```python
from build123d import *

# Parameters (mm, degrees)
EXTRUDE_1_DEPTH          = 3
EXTRUDE_2_DEPTH          = 287
SKETCH_4_W               = 21.736589458
SKETCH_4_H               = 200
CUT_EXTRUDE_1_DEPTH      = 43
SKETCH_5_W               = 23.415155123
SKETCH_5_H               = 200
CUT_EXTRUDE_2_DEPTH      = 43
CUT_EXTRUDE_6_DEPTH      = 100
CUT_EXTRUDE_6_DEPTH_BACK = 100
SKETCH_6_W               = 303.843563536
SKETCH_6_H               = 206
HOLE_WIZARD_1_AT_2_COUNT = 2
HOLE_WIZARD_1_AT_2_PITCH = 10
HOLE_WIZARD_1_AT_3_COUNT = 2
HOLE_WIZARD_1_AT_3_PITCH = 31.622776602
HOLE_WIZARD_1_AT_4_COUNT = 2
HOLE_WIZARD_1_AT_4_PITCH = 30
CUT_EXTRUDE_7_DEPTH      = 30


with BuildPart() as part:
    # 草图1 → 凸台-拉伸1 (new body)
    with BuildSketch(Plane.XY):
        Polygon((-143.75, 30), (-143.75, 70), (-105.75, 70), (-105.75, 65), (-100.25, 65), (-100.25, 70), (99.75, 70), (99.75, 65), (105.25, 65), (105.25, 70), (143.25, 70), (143.25, 30), (135.25, 30), (135.25, -30), (143.25, -30), (143.25, -70), (105.25, -70), (105.25, -65), (99.75, -65), (99.75, -70), (-100.25, -70), (-100.25, -65), (-105.75, -65), (-105.75, -70), (-143.75, -70), (-143.75, -30), (-135.75, -30), (-135.75, 30), align=None)
    extrude(amount=EXTRUDE_1_DEPTH)

    # 草图2 → 凸台-拉伸2 (add)
    with BuildSketch(Plane.ZY.offset(143.75)):
        with BuildLine():
            Line((0, 70), (0, 30))
            Line((0, 30), (-3, 33))
            Line((-3, 33), (-3, 70))
            ThreePointArc((-3, 70), (6.665476221, 93.334523779), (30, 103))
            Line((30, 103), (47, 103))
            Line((47, 103), (50, 100))
            Line((50, 100), (45, 90))
            Line((45, 90), (60, 90))
            Line((60, 90), (60, 87))
            Line((60, 87), (41, 87))
            Line((41, 87), (47, 100))
            Line((47, 100), (30, 100))
            ThreePointArc((30, 100), (8.786796564, 91.213203436), (0, 70))
        make_face()
        with BuildLine():
            Line((30, -100), (47, -100))
            Line((47, -100), (41, -87))
            Line((41, -87), (60, -87))
            Line((60, -87), (60, -90))
            Line((60, -90), (45, -90))
            Line((45, -90), (50, -100))
            Line((50, -100), (47, -103))
            Line((47, -103), (30, -103))
            ThreePointArc((30, -103), (6.665476221, -93.334523779), (-3, -70))
            Line((-3, -70), (-3, -33))
            Line((-3, -33), (0, -30))
            Line((0, -30), (0, -70))
            ThreePointArc((0, -70), (8.786796564, -91.213203436), (30, -100))
        make_face()
    extrude(amount=-EXTRUDE_2_DEPTH)

    # 草图4 → 切除-拉伸1 (cut)
    with BuildSketch(Plane.ZY.offset(143.75)):
        with Locations((49.368294729, 0)):
            Rectangle(SKETCH_4_W, SKETCH_4_H)
    extrude(amount=-CUT_EXTRUDE_1_DEPTH, mode=Mode.SUBTRACT)

    # 草图5 → 切除-拉伸2 (cut)
    with BuildSketch(Plane(origin=(143.25, 0, 0), x_dir=(0, 0, -1), z_dir=(1, 0, 0))):
        with Locations((-51.459603014, 0)):
            Rectangle(SKETCH_5_W, SKETCH_5_H)
    extrude(amount=-CUT_EXTRUDE_2_DEPTH, mode=Mode.SUBTRACT)

    # 草图6 → 切除-拉伸6 (cut, two sides: drawn at the far end of the back side and taken through both)
    with BuildSketch(Plane.XY.offset(-CUT_EXTRUDE_6_DEPTH_BACK)):
        with Locations((51.171781768, 0)):
            Rectangle(SKETCH_6_W, SKETCH_6_H)
    extrude(amount=CUT_EXTRUDE_6_DEPTH + CUT_EXTRUDE_6_DEPTH_BACK, mode=Mode.SUBTRACT)

    # 草图8 → 大小六角凹头盖螺钉柱孔1 (revolve, cut)
    with BuildSketch(Plane(origin=(-115.75, 15, 0), x_dir=(0, 1, 0), z_dir=(1, 0, 0))):
        Polygon((0, 0), (0, 50), (1.2, 50), (1.2, 2), (2.15, 2), (2.15, 0.024142219), (2.175, 0), align=None)
    hole_wizard_1 = revolve(axis=Axis((-115.75, 15, -6.35), (0, 0, 1)), mode=Mode.SUBTRACT)

    # 大小六角凹头盖螺钉柱孔1 at 2: 大小六角凹头盖螺钉柱孔1 ×2
    with Locations(*[(-i * HOLE_WIZARD_1_AT_2_PITCH, 0, 0) for i in range(1, HOLE_WIZARD_1_AT_2_COUNT)]):
        add(hole_wizard_1, mode=Mode.SUBTRACT)

    # 大小六角凹头盖螺钉柱孔1 at 3: 大小六角凹头盖螺钉柱孔1 ×2
    with Locations(*[Vector(-0.3162277660168408, -0.9486832980505129, 0) * (i * HOLE_WIZARD_1_AT_3_PITCH) for i in range(1, HOLE_WIZARD_1_AT_3_COUNT)]):
        add(hole_wizard_1, mode=Mode.SUBTRACT)

    # 大小六角凹头盖螺钉柱孔1 at 4: 大小六角凹头盖螺钉柱孔1 ×2
    with Locations(*[(0, -i * HOLE_WIZARD_1_AT_4_PITCH, 0) for i in range(1, HOLE_WIZARD_1_AT_4_COUNT)]):
        add(hole_wizard_1, mode=Mode.SUBTRACT)

    # 草图10 → 切除-拉伸7 (cut)
    with BuildSketch(Plane.ZY.offset(135.75)):
        with BuildLine():
            Line((30, 100), (47, 100))
            Line((47, 100), (45.5, 101.5))
            Line((45.5, 101.5), (30, 101.5))
            ThreePointArc((30, 101.5), (7.726136393, 92.273863607), (-1.5, 70))
            Line((-1.5, 70), (-1.5, 37.5))
            Line((-1.5, 37.5), (3, 33))
            Line((3, 33), (3, 70))
            Line((3, 70), (0, 70))
            ThreePointArc((0, 70), (8.786796564, 91.213203436), (30, 100))
        make_face()
        with BuildLine():
            Line((-1.5, -37.5), (-1.5, -70))
            ThreePointArc((-1.5, -70), (7.726136393, -92.273863607), (30, -101.5))
            Line((30, -101.5), (45.5, -101.5))
            Line((45.5, -101.5), (47, -100))
            Line((47, -100), (30, -100))
            ThreePointArc((30, -100), (8.786796564, -91.213203436), (0, -70))
            Line((0, -70), (3, -70))
            Line((3, -70), (3, -33))
            Line((3, -33), (-1.5, -37.5))
        make_face()
    extrude(amount=-CUT_EXTRUDE_7_DEPTH, mode=Mode.SUBTRACT)


solid = part.part
```
Geometry check sheet. Reference: the model listing, model coordinates, mm. A direction names the side the tool comes from. Round coordinates to 2 decimals unless told otherwise and drop trailing zeros. Write each loop counter-clockwise with the first axis right and the second up, starting at its lowest first coordinate (ties: lowest second). Pieces come first, ordered by that corner, then holes. Notation, with made-up numbers: (20, 81) -> (55, 81) arc R23 cw to (55, 119) -> close; hole circle Ø4 at (-1.75, 64). An arc over 180 degrees is marked (long way). Put each result on its own line as item: value.
1) Release check for a two-part mould opening along X. For faces 1 (the face through (-103, 68, 0)), 2 (the face through (-114, -15, 2)), 3 (the face through (-143.75, 69, 2)) record: pulls with the +X half, pulls with the -X half, needs draft (parallel to the pull), parting line crosses it, or undercut.
Recorded:
face 1: needs draft
face 2: undercut
face 3: pulls with the -X half
2) Thickness scan on probe 1 along X at (y, z) = (-15, 2.45); probe 2 along X at (y, z) = (15, 1.25); probe 3 along Y at (x, z) = (-120, 43.5). Record the ranges inside material, lowest first. Write a range as from..to.
Recorded:
probe 1: x = -135.75..-126.95, -124.55..-116.95, -114.55..-100.75
probe 2: x = -135.75..-127.9, -123.6..-117.9, -113.6..-100.75
probe 3: y = -103..-101.5, 101.5..103
3) Cross-section at B-B, the plane z = 35. Enter the section's corners in (x, y).
Recorded:
outline: (-143.75, -103) -> (-100.75, -103) -> (-100.75, -100) -> (-105.75, -100) -> (-105.75, -101.5) -> (-135.75, -101.5) -> (-135.75, -100) -> (-143.75, -100) -> close; (-143.75, 100) -> (-135.75, 100) -> (-135.75, 101.5) -> (-105.75, 101.5) -> (-105.75, 100) -> (-100.75, 100) -> (-100.75, 103) -> (-143.75, 103) -> close
4) Depth check by flat-ended pin: P1, Ø3.5, axis at x = -125.75, y = -15, coming from the +Z side; P2, Ø8, axis at x = -122.5, z = 23.5, coming from the -Y side; P3, Ø7, axis at x = -125.75, y = 15, coming from the -Z side; P4, Ø6, axis at y = -81.5, z = 7, coming from the -X side. Enter the tip coordinate at first touch or a pass-through.
Recorded:
P1: stops at z = 3
P2: stops at y = -102.91
P3: stops at z = 0
P4: passes through
5) Cross-section at A-A, the plane x = -139. Enter the section's corners in (y, z), plus the area to 3 significant figures.
Recorded:
outline: (-103, 30) arc R33 ccw to (-70, -3) -> (-33, -3) -> (-30, 0) -> (-30, 3) -> (-70, 3) -> (-70, 0) arc R30 cw to (-100, 30) -> (-100, 50) -> (-103, 47) -> close; (30, 0) -> (33, -3) -> (70, -3) arc R33 ccw to (103, 30) -> (103, 47) -> (100, 50) -> (100, 30) arc R30 cw to (70, 0) -> (70, 3) -> (30, 3) -> close
area: 879 mm2
6) Access from +Z, -Z, +X, -X, +Y, -Y to the whole of each face (thin tool, end or side, straight path). Record for faces 4 (the face through (-122.551, 93.077, 6.41)), 5 (the face through (-135.75, 67, 1)), 6 (the face through (-139.806, -90.979, 8.555)), 7 (the face through (-123.65, -15.47, 1)), 8 (the face through (-121, -54, -1.5)).
Recorded:
face 4: -Z, +X, -X, +Y
face 5: none
face 6: +Z, +X, -X
face 7: -Z
face 8: +Z
7) Cross-section at C-C, the plane z = 18. Enter the section's corners in (x, y).
Recorded:
outline: (-143.75, -100.74) -> (-100.75, -100.74) -> (-100.75, -97.5) -> (-105.75, -97.5) -> (-105.75, -99.12) -> (-135.75, -99.12) -> (-135.75, -97.5) -> (-143.75, -97.5) -> close; (-143.75, 97.5) -> (-135.75, 97.5) -> (-135.75, 99.12) -> (-105.75, 99.12) -> (-105.75, 97.5) -> (-100.75, 97.5) -> (-100.75, 100.74) -> (-143.75, 100.74) -> close
8) Cross-section at D-D, the plane y = 19.5. Enter the section's corners in (x, z), plus the area to 3 significant figures.
Recorded:
outline: (-135.75, 0) -> (-100.75, 0) -> (-100.75, 3) -> (-135.75, 3) -> close
area: 105 mm2
